Check sheet for the drawn part. Datum: minimum x, y, z corner. Units: mm. Coordinates: 2 decimals unless noted, no trailing zeros. One line per question, with ' | ' between items.
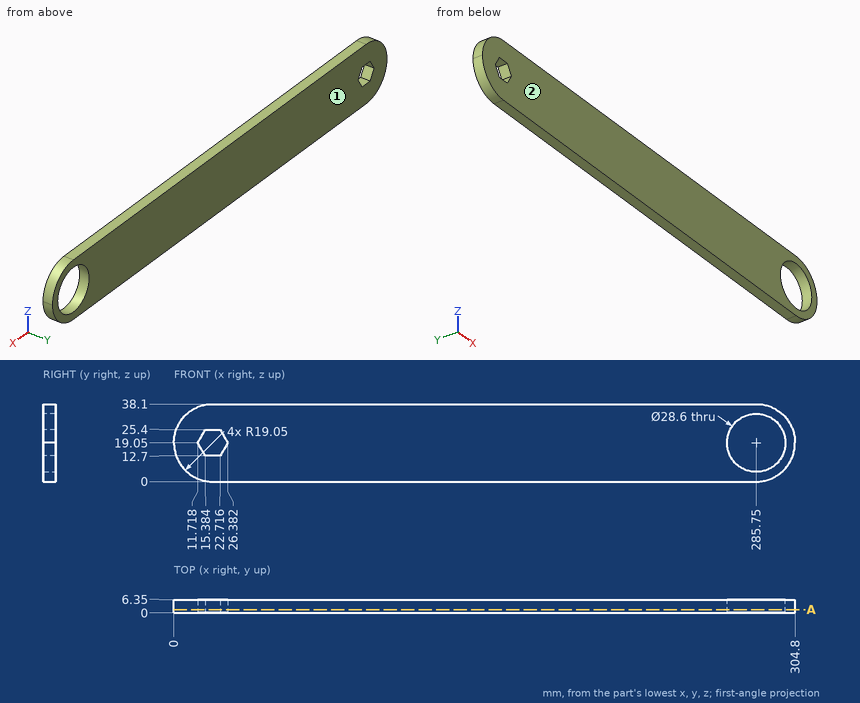
1. Mould release check, pull along Y, two halves, no side actions. Record for the marked faces 1 and 2: released by +Y, released by -Y, zero draft, split by the parting line, or undercut.
Worked answers:
face 1: released by +Y | face 2: released by -Y
2. Cross-section at A-A on y = 1.5. Give the number of separate pieces and of enclosed holes in the cut face, and give its area (3 significant figures).
Worked answers:
separate pieces: 1 | enclosed holes: 2 | area: 10,500 mm²
3. Go/stop test with a flat-tipped pin: P1, Ø1.5, axis at y = 2.5, z = 23.5, coming from the +X side. Record where the tip stops, or that it passes through.
Worked answers:
P1: x = 304.44
4. Material ranges on line 1 (X direction, y = 4, z = 14) (1 decimal); line 2 (X direction, y = 4, z = 31) (1 decimal); line 3 (X direction, y = 1.5, z = 29) (1 decimal), recorded low to high. Write a range as from..to.
Worked answers:
line 1: 0.7..14.6, 23.5..272.4, 299.1..304.1 | line 2: 4.2..277.9, 293.6..300.6 | line 3: 2.8..275.5, 296..302
